from build123d import *

# Parameters (mm, degrees)
SKETCH_1_R           = 18.5
SKETCH_1_R_2         = 13.5
EXTRUDE_1_DEPTH      = 10
EXTRUDE_2_REACH      = 145.054
EXTRUDE_2_END_RADIUS = 18.5
SKETCH_3_R           = 10
SKETCH_4_W           = 30
SKETCH_4_H           = 30
EXTRUDE_3_DEPTH      = 15
SKETCH_5_R           = 2
CUT_EXTRUDE_1_DEPTH  = 15
SKETCH_6_R           = 4.5
CUT_EXTRUDE_2_DEPTH  = 1.5


with BuildPart() as part:
    # 草图1 → 凸台-拉伸1 (new, symmetric)
    with BuildSketch(Plane.XY):
        Circle(SKETCH_1_R)
        Circle(SKETCH_1_R_2, mode=Mode.SUBTRACT)
    extrude(amount=EXTRUDE_1_DEPTH, both=True)

    # 凸台-拉伸2: up to this cylinder (the profile starts outside it)
    extrude_2_end = Plane(origin=(0, 0, 0), z_dir=(0, 0, -1)) * Cylinder(EXTRUDE_2_END_RADIUS, 328.108, mode=Mode.PRIVATE)
    # 草图3 → 凸台-拉伸2 (add, up to the surface)
    with BuildSketch(Plane(origin=(0, 123, 0), x_dir=(1, 0, 0), z_dir=(0, 1, 0)), mode=Mode.PRIVATE) as extrude_2_sk1:
        with Locations(Location((0, 0, 0), (0, 0, 270))):
            Circle(SKETCH_3_R)
    extrude_2_tool1 = extrude(extrude_2_sk1.sketch, amount=-EXTRUDE_2_REACH, mode=Mode.PRIVATE) - extrude_2_end
    add(extrude_2_tool1.solids().sort_by_distance((0, 123, 0))[0])

    # 草图4 → 凸台-拉伸3 (add)
    with BuildSketch(Plane(origin=(0, 123, 0), x_dir=(1, 0, 0), z_dir=(0, 1, 0))):
        Rectangle(SKETCH_4_W, SKETCH_4_H)
    extrude(amount=EXTRUDE_3_DEPTH)

    # 草图5 → 切除-拉伸1 (cut)
    with BuildSketch(Plane(origin=(0, 138, 0), x_dir=(1, 0, 0), z_dir=(0, 1, 0))):
        with Locations(Location((-10, 10, 0), (0, 0, 270))):
            Circle(SKETCH_5_R)
        with Locations(Location((10, 10, 0), (0, 0, 270))):
            Circle(SKETCH_5_R)
        with Locations(Location((-10, -10, 0), (0, 0, 270))):
            Circle(SKETCH_5_R)
        with Locations(Location((10, -10, 0), (0, 0, 270))):
            Circle(SKETCH_5_R)
    extrude(amount=-CUT_EXTRUDE_1_DEPTH, mode=Mode.SUBTRACT)

    # 草图6 → 切除-拉伸2 (cut)
    with BuildSketch(Plane.XZ.offset(-123)):
        with Locations(Location((-10, -10, 0), (0, 0, 270))):
            Circle(SKETCH_6_R)
        with Locations(Location((-10, 10, 0), (0, 0, 270))):
            Circle(SKETCH_6_R)
        with Locations(Location((10, 10, 0), (0, 0, 270))):
            Circle(SKETCH_6_R)
        with Locations(Location((10, -10, 0), (0, 0, 270))):
            Circle(SKETCH_6_R)
    extrude(amount=-CUT_EXTRUDE_2_DEPTH, mode=Mode.SUBTRACT)


solid = part.part
Geometry: final body of the model. Coordinates: model frame, mm. A direction names the side the tool comes from. Coordinates: 2 decimals unless noted, no trailing zeros. Order: outer loops, then holes, each group sorted by start corner. A loop starts at its lowest first (then second) coordinate and runs counter-clockwise, first axis right, second up.
(1) First-contact query: pin 1 (6 mm diameter, centred on x = -7.5, z = -9.5, fed in from -Y); pin 2 (7.5 mm diameter, centred on y = 132.5, z = -5, fed in from -X); pin 3 (5.5 mm diameter, centred on x = -10, z = -10, fed in from -Y). Flat tips, straight axial feed; report the tip coordinate or a pass-through.
(2) Section query A-A (y = 0). Return the cut outline in (x, z), plus the area to 3 significant figures.
(3) Access query for faces 4 (the face through (-8.648, 123.74, 5.708)), 5 (the face through (-8, 131, 10)), 6 (the face through (15, 130, 0)), 7 (the face through (0, 130, 15)). Directions: +Z, -Z, +X, -X, +Y, -Y. A direction counts if a zero-diameter tool reaches every point of the face in a straight line with its end or side. Return the directions, or none.
(4) Section query B-B (y = 118). Return the cut outline in (x, z), plus the area to 3 significant figures.
(5) Material intervals for probe 1 along Z at (x, y) = (10, 123.9); probe 2 along X at (y, z) = (133.75, 10), sorted ascending.
(6) Draft query along X for faces 1 (the face through (-11, 124.5, 8)), 2 (the face through (1, -14, -10)), 3 (the face through (-9.76, 70.03, -2.17)). Return one class per face: pulls with the +X half, pulls with the -X half, needs draft (parallel to the pull), parting line crosses it, or undercut.
Solution:
1. pin 1: stops at y = -17.94
1. pin 2: stops at x = -15
1. pin 3: stops at y = -17.02
2. outline: (-18.5, -10) - (-13.5, -10) - (-13.5, 10) - (-18.5, 10) - close; (13.5, -10) - (18.5, -10) - (18.5, 10) - (13.5, 10) - close
2. area: 200 mm2
3. face 4: none
3. face 5: +Y
3. face 6: +Z, -Z, +X, +Y
3. face 7: +Z, +X, -X, +Y, -Y
4. outline: circle Ø20 at (0, 0)
4. area: 314 mm2
5. probe 1: z = -15 to -14.5, -5.5 to 5.5, 14.5 to 15
5. probe 2: x = -15 to -12, -8 to 8, 12 to 15
6. face 1: undercut
6. face 2: needs draft
6. face 3: parting line crosses it
